from build123d import *

# Parameters (mm, degrees)
CUT_EXTRUDE1_DEPTH = 22.7
SKETCH3_R          = 1.6
CUT_EXTRUDE2_DEPTH = 6
CIRPATTERN1_COUNT  = 4


with BuildPart() as part:
    # Sketch1 → Revolve1 (revolve)
    with BuildSketch(Plane.XY):
        with BuildLine():
            Line((0, 188.999977867), (0, 201.699977867))
            Line((0, 201.699977867), (-3, 201.699977867))
            Line((-3, 201.699977867), (-3, 188.999977867))
            Line((-3, 188.999977867), (-8, 188.999977867))
            Line((-8, 188.999977867), (0.570207018, 178.999977867))
            add(Edge.make_bspline(
                [(-3, 19.999977867), (17.518474446, 71.927932429), (18.708543453, 124.927932429), (0.570207018, 178.999977867)],
                knots=[0, 0, 0, 0, 0.942000122, 0.942000122, 0.942000122, 0.942000122], degree=3))
            Line((-3, 19.999977867), (-8, 19.999977867))
            Line((-8, 19.999977867), (-8, -30.000022133))
            Line((-8, -30.000022133), (-3, -30.000022133))
            Line((-3, -30.000022133), (-3, -42.700022133))
            Line((-3, -42.700022133), (0, -42.700022133))
            Line((0, -42.700022133), (0, -30.000022133))
            Line((0, -30.000022133), (0, 20.000038989))
            add(Edge.make_bspline(
                [(0, 20.000038989), (32.67273479, 102.687818928), (0, 188.999977867)],
                knots=[0, 0, 0, 1, 1, 1], degree=2))
        make_face()
    revolve(axis=Axis((37.402673701, -40.000005834, 0), (0, 1, 0)))

    # Sketch2 → Cut-Extrude1 (cut)
    with BuildSketch(Plane.XZ.offset(42.700022133)):
        with BuildLine():
            Line((25.405862227, 5), (-3, 5))
            Line((-3, 5), (-3, -5))
            Line((-3, -5), (25.405862227, -5))
            ThreePointArc((25.405862227, -5), (28.2123667, -9.190307001), (32.402673701, -11.996811474))
            Line((32.402673701, -11.996811474), (32.402673701, -40.402673701))
            Line((32.402673701, -40.402673701), (42.402673701, -40.402673701))
            Line((42.402673701, -40.402673701), (42.402673701, -11.996811474))
            ThreePointArc((42.402673701, -11.996811474), (46.592980702, -9.190307001), (49.399485175, -5))
            Line((49.399485175, -5), (77.805347402, -5))
            Line((77.805347402, -5), (77.805347402, 5))
            Line((77.805347402, 5), (49.399485175, 5))
            ThreePointArc((49.399485175, 5), (46.592980702, 9.190307001), (42.402673701, 11.996811474))
            Line((42.402673701, 11.996811474), (42.402673701, 40.402673701))
            Line((42.402673701, 40.402673701), (32.402673701, 40.402673701))
            Line((32.402673701, 40.402673701), (32.402673701, 11.996811474))
            ThreePointArc((32.402673701, 11.996811474), (28.2123667, 9.190307001), (25.405862227, 5))
        make_face()
    extrude(amount=-CUT_EXTRUDE1_DEPTH, mode=Mode.SUBTRACT)

    # Sketch3 → Cut-Extrude2 (cut, through all)
    with BuildSketch(Plane(origin=(-3, 0, 0), x_dir=(0, 0, -1), z_dir=(1, 0, 0))):
        with Locations((0, -25.000022133)):
            Circle(SKETCH3_R)
    cut_extrude2 = extrude(amount=-CUT_EXTRUDE2_DEPTH, mode=Mode.SUBTRACT)

    # CirPattern1: Cut-Extrude2 ×4 about axis
    cirpattern1_axis = Axis((37.402673701, 20.000038989, 0), (0, -1, 0))
    for i in range(1, CIRPATTERN1_COUNT):
        add(cut_extrude2.rotate(cirpattern1_axis, i * 360 / CIRPATTERN1_COUNT), mode=Mode.SUBTRACT)


solid = part.part
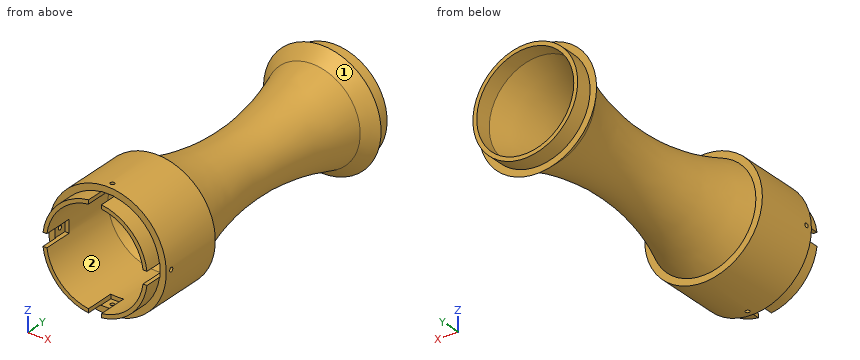
Geometry check sheet. Reference: the model listing, model coordinates, mm. Face numbers are marked on the shaded views. Round coordinates to 2 decimals unless told otherwise and drop trailing zeros. One line per item, written item: value. Start each with the question number.
(1) Draft check along Z on the marked faces 1 and 2. Enter one of: +Z half, -Z half, draft (parallel to the pull), parting line (faces both ways), or undercut.
(2) Go/stop test with flat-tipped pins: pin 1 Ø8 at (y, z) = (21, -20) entering from +X; pin 2 Ø5 at (y, z) = (102, -17.5) entering from +X; pin 3 Ø2 at (x, y) = (32, 4) entering from -Z; pin 4 Ø2.5 at (y, z) = (-25, 0) entering from +X. Record where each tip stops, or that it passes through.
(3) Scan lines: line 1 (Z direction, x = 42, y = 27); line 2 (Y direction, x = -4.7, z = 0); line 3 (Z direction, x = 24, y = 158.5). Record each from-to range of solid material in increasing order. Write a range as [from, to].
Answer:
1. face 1: parting line
1. face 2: undercut
2. pin 1: x = 79.84
2. pin 2: x = 56.23
2. pin 3: z = -45.19
2. pin 4: through
3. line 1: [-37.48, -34.45], [34.45, 37.48]
3. line 2: [-30, -26.6], [-23.4, 20], [185.15, 189]
3. line 3: [-27.81, -24.43], [24.43, 27.81]
